Work out the finished part from the listing and answer in its coordinate system (mm). Coordinates: 2 decimals unless noted, no trailing zeros. Loops run counter-clockwise (first coordinate to the right, second up) from the corner with the lowest first, then second, coordinate; pieces in that order, holes last. Notation, with made-up numbers: (65, -36.5) -> (81, -36.5) arc R38 ccw to (81, 2.5) -> close; hole circle Ø5 at (-4, -35). An arc over 180 degrees is marked (long way). One line per question, with ' | ' between items.
```python
from build123d import *

# Parameters (mm, degrees)
ESBO_O1_R                = 0.8
RESSALTO_EXTRUS_O1_DEPTH = 3
FILETE1_R                = 3
FILETE2_R                = 3


with BuildPart() as part:
    # Esboço1 → Ressalto-extrusão1 (new body)
    with BuildSketch(Plane(origin=(0, 0, 0), x_dir=(0, 0, -1), z_dir=(1, 0, 0))):
        with BuildLine():
            Line((-26.317877539, 0), (-26.317877539, 7.5))
            Line((-26.317877539, 7.5), (8.682122461, 7.5))
            Line((8.682122461, 7.5), (36.475999374, 1.826598632))
            ThreePointArc((36.475999374, 1.826598632), (37.625192713, 1.131917902), (38.075999374, -0.132993162))
            Line((38.075999374, -0.132993162), (38.075999374, -1.030306154))
            ThreePointArc((38.075999374, -1.030306154), (37.599230732, -2.326364112), (36.396233145, -3.004502277))
            Line((36.396233145, -3.004502277), (8.682122461, -7.5))
            Line((8.682122461, -7.5), (-26.317877539, -7.5))
            Line((-26.317877539, -7.5), (-26.317877539, 0))
        make_face()
        with Locations((-23.317877539, 4.5)):
            Circle(ESBO_O1_R, mode=Mode.SUBTRACT)
        with Locations((5.682122461, -4.5)):
            Circle(ESBO_O1_R, mode=Mode.SUBTRACT)
        with Locations((35.075999374, -0.719592125)):
            Circle(ESBO_O1_R, mode=Mode.SUBTRACT)
    extrude(amount=RESSALTO_EXTRUS_O1_DEPTH)

    # Filete1
    filete1_edges = [part.edges().sort_by_distance(p)[0] for p in [
        (1.5, -7.5, 26.317877539),
    ]]
    fillet(filete1_edges, radius=FILETE1_R)

    # Filete2
    filete2_edges = [part.edges().sort_by_distance(p)[0] for p in [
        (1.5, 7.5, 26.317877539),
    ]]
    fillet(filete2_edges, radius=FILETE2_R)


solid = part.part
```
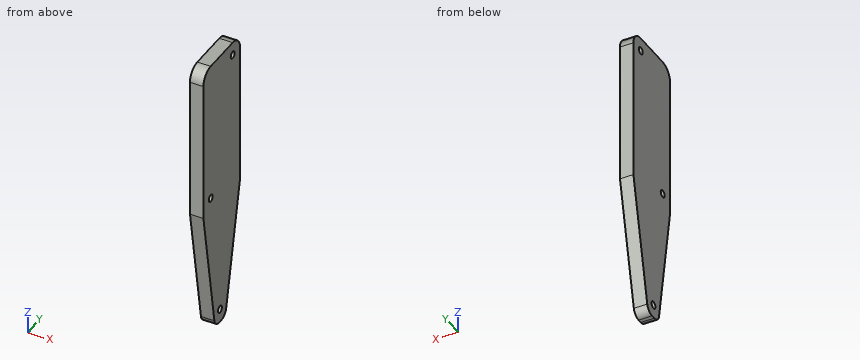
1) Find section B-B (y = -6.25). Write down the section's boundary in (x, z), plus the area to 3 significant figures.
Check values:
outline: (0, -16.39) -> (3, -16.39) -> (3, 25.75) -> (0, 25.75) -> close | area: 126 mm^2
2) Find section A-A (x = 1.8). Write down the section's boundary in (y, z), plus the area to 3 significant figures.
Check values:
outline: (-7.5, -8.68) -> (-3, -36.4) arc R2 ccw to (-1.03, -38.08) -> (-0.13, -38.08) arc R2 ccw to (1.83, -36.48) -> (7.5, -8.68) -> (7.5, 23.32) arc R3 ccw to (4.5, 26.32) -> (-4.5, 26.32) arc R3 ccw to (-7.5, 23.32) -> close; hole circle Ø1.6 at (-4.5, -5.68); hole circle Ø1.6 at (-0.72, -35.08); hole circle Ø1.6 at (4.5, 23.32) | area: 797 mm^2
3) Find section C-C (z = -14.5). Write down the section's boundary in (x, y).
Check values:
outline: (0, -6.56) -> (3, -6.56) -> (3, 6.31) -> (0, 6.31) -> close
4) Find the intervals of material crossed by line 1 along Z through (x, y) = (0.55, -0.5); line 2 along Y through (x, z) = (0.75, -12); line 3 along Y through (x, z) = (1.25, -25), in increasing order.
Check values:
line 1: z = -38.08 to -35.85, -34.31 to 26.32 | line 2: y = -6.96 to 6.82 | line 3: y = -4.85 to 4.17
5) Flat-ended cylindrical pins translate along their axes: pin 1 (1.3 mm diameter, centred on y = 4.5, z = 23.32, fed in from -X); pin 2 (2.5 mm diameter, centred on y = -4.5, z = -5.68, fed in from +X). Find the tip coordinate at first contact, or state that the pin passes through.
Check values:
pin 1: passes through | pin 2: stops at x = 3
